Here's how the part is built. I have some questions about the finished solid (model axes, mm). A direction names the side the tool comes from. Coordinates: 2 decimals unless noted, no trailing zeros. Order: outer loops, then holes, each group sorted by start corner. A loop starts at its lowest first (then second) coordinate and runs counter-clockwise, first axis right, second up.
```python
from build123d import *

# Parameters (mm, degrees)
SKETCH1_R                                      = 17.5
BOSS_EXTRUDE1_DEPTH                            = 1.5
CUT_EXTRUDE1_DEPTH                             = 25.794152536
CUT_EXTRUDE1_DEPTH_BACK                        = 25.794152536
SKETCH6_R                                      = 0.25
SKETCH6_R_2                                    = 1
CBORE_FOR_0_SOCKET_HEAD_CAP_SCREW1_D           = 1.778
CBORE_FOR_0_SOCKET_HEAD_CAP_SCREW1_CBORE_D     = 3.175
CBORE_FOR_0_SOCKET_HEAD_CAP_SCREW1_CBORE_DEPTH = 1.016
BOSS_EXTRUDE2_START                            = -1.5
BOSS_EXTRUDE2_DEPTH                            = 1.5
FILLET1_DEPTH                                  = 1.5
CUT_EXTRUDE2_START                             = -10
SKETCH16_R                                     = 1
CUT_EXTRUDE2_DEPTH                             = 10
SKETCH17_R                                     = 6.9
CUT_EXTRUDE3_DEPTH                             = 1
FILLET2_R                                      = 0.5


with BuildPart() as part:
    # Sketch1 → Boss-Extrude1 (new body)
    with BuildSketch(Plane(origin=(0, 0, 0), x_dir=(1, 0, 0), z_dir=(0, 1, 0))):
        with Locations(Location((0, 0, 0), (0, 0, 270))):
            Circle(SKETCH1_R)
    extrude(amount=BOSS_EXTRUDE1_DEPTH)

    # Sketch6 → Cut-Extrude1 (cut, two sides: drawn at the far end of the back side and taken through both)
    with BuildSketch(Plane(origin=(0, 1.5, 0), x_dir=(1, 0, 0), z_dir=(0, 1, 0)).offset(-CUT_EXTRUDE1_DEPTH_BACK)):
        with Locations(Location((0, 12.5, 0), (0, 0, 270))):
            Circle(SKETCH6_R)
        with Locations(Location((11.591109915, 3.105828541, 0), (0, 0, 270))):
            Circle(SKETCH6_R_2)
    extrude(amount=CUT_EXTRUDE1_DEPTH + CUT_EXTRUDE1_DEPTH_BACK, mode=Mode.SUBTRACT)

    # CBORE for #0 Socket Head Cap Screw1 (through all)
    with Locations(Plane(origin=(0, 1.5, 0), x_dir=(1, 0, 0), z_dir=(0, 1, 0))):
        with Locations((0, 15), (-15, 0), (0, -15), (15, 0)):
            CounterBoreHole(CBORE_FOR_0_SOCKET_HEAD_CAP_SCREW1_D / 2, CBORE_FOR_0_SOCKET_HEAD_CAP_SCREW1_CBORE_D / 2, CBORE_FOR_0_SOCKET_HEAD_CAP_SCREW1_CBORE_DEPTH)

    # Sketch15 → Boss-Extrude2 (add)
    # profile 1 of 3: a face of its own
    with BuildSketch(Plane(origin=(0, 1.5, 0), x_dir=(1, 0, 0), z_dir=(0, 1, 0)).offset(BOSS_EXTRUDE2_START)):
        with BuildLine():
            ThreePointArc((-5.176050603, 16.717012297), (-4.139884011, 17.00327499), (-3.0880962, 17.225378424))
            Line((-3.0880962, 17.225378424), (-3.2615852, 17.702035532))
            ThreePointArc((-3.2615852, 17.702035532), (-7.18242301, 19.733545037), (-8.880129888, 15.657052506))
            ThreePointArc((-8.880129888, 15.657052506), (-8.884731942, 15.654441488), (-8.889333228, 15.651829119))
            Line((-8.889333228, 15.651829119), (-8.715826512, 15.175123334))
            ThreePointArc((-8.715826512, 15.175123334), (-7.762905696, 15.68398212), (-6.780403574, 16.133075571))
            ThreePointArc((-6.780403574, 16.133075571), (-6.498382723, 17.854159795), (-5.176050603, 16.717012297))
        make_face()
    # profile 2 of 3: a face of its own
    with BuildSketch(Plane(origin=(0, 1.5, 0), x_dir=(1, 0, 0), z_dir=(0, 1, 0)).offset(BOSS_EXTRUDE2_START)):
        with BuildLine():
            ThreePointArc((17.242700391, 2.989863415), (17.499999999, 0.00015134), (17.242752101, -2.989565186))
            Line((17.242752101, -2.989565186), (17.75, -2.989565186))
            ThreePointArc((17.75, -2.989565186), (21, 0), (17.75, 2.989565186))
            Line((17.75, 2.989565186), (17.242700391, 2.989863415))
        make_face()
        with BuildLine():
            ThreePointArc((17.972222222, 0.999614123), (19, 0), (17.972222222, -0.999614123))
            ThreePointArc((17.972222222, -0.999614123), (18, 0), (17.972222222, 0.999614123))
        make_face(mode=Mode.SUBTRACT)
    # profile 3 of 3: a face of its own
    with BuildSketch(Plane(origin=(0, 1.5, 0), x_dir=(1, 0, 0), z_dir=(0, 1, 0)).offset(BOSS_EXTRUDE2_START)):
        with BuildLine():
            ThreePointArc((-8.880129888, -15.657052506), (-6.943930938, -19.809244554), (-3.170985611, -17.210312323))
            ThreePointArc((-3.170985611, -17.210312323), (-4.180800117, -16.993260734), (-5.176050603, -16.717012297))
            ThreePointArc((-5.176050603, -16.717012297), (-6.498382723, -17.854159795), (-6.780403574, -16.133075571))
            ThreePointArc((-6.780403574, -16.133075571), (-7.758295007, -15.686263372), (-8.706903461, -15.180244798))
            Line((-8.706903461, -15.180244798), (-8.880129888, -15.657052506))
        make_face()
    extrude(amount=BOSS_EXTRUDE2_DEPTH)

    # Fillet1: read off the stored shape, not the designer's step
    # Fillet1 outline → Fillet1 (add)
    with BuildSketch(Plane(origin=(0, 0, 0), x_dir=(1, 0, 0), z_dir=(0, 1, 0))):
        with BuildLine():
            ThreePointArc((-8.889333228, 15.651829119), (-9.197952649, 15.040582781), (-9.694667487, 14.56926293))
            ThreePointArc((-9.694667487, 14.56926293), (-9.210230129, 14.880243982), (-8.715826512, 15.175123334))
            Line((-8.715826512, 15.175123334), (-8.889333228, 15.651829119))
        make_face()
        with BuildLine():
            ThreePointArc((-9.943920594, -14.400293164), (-9.235099699, -15.274689897), (-9.110766229, -16.393411442))
            ThreePointArc((-9.110766229, -16.393411442), (-9.019221723, -16.017785781), (-8.880129888, -15.657052506))
            Line((-8.880129888, -15.657052506), (-8.706903461, -15.180244798))
            ThreePointArc((-8.706903461, -15.180244798), (-9.33356259, -14.803195918), (-9.943920594, -14.400293164))
        make_face()
        with BuildLine():
            ThreePointArc((-3.0880962, 17.225378424), (-2.365537121, 17.339383902), (-1.638844908, 17.423093507))
            ThreePointArc((-1.638844908, 17.423093507), (-2.743884601, 17.637298977), (-3.558229913, 18.414369386))
            ThreePointArc((-3.558229913, 18.414369386), (-3.386909552, 18.067779761), (-3.2615852, 17.702035532))
            Line((-3.2615852, 17.702035532), (-3.0880962, 17.225378424))
        make_face()
        with BuildLine():
            ThreePointArc((17.75, 2.989565186), (18.136550606, 2.996890711), (18.520833333, 2.954442865))
            ThreePointArc((18.520833333, 2.954442865), (17.512103504, 3.453903412), (16.93287037, 4.419038472))
            ThreePointArc((16.93287037, 4.419038472), (17.102720385, 3.707688694), (17.242700391, 2.989863415))
            Line((17.242700391, 2.989863415), (17.75, 2.989565186))
        make_face()
        with BuildLine():
            ThreePointArc((17.242752101, -2.989565186), (17.102752448, -3.70754079), (16.932870371, -4.419038472))
            ThreePointArc((16.932870371, -4.419038472), (17.512103504, -3.453903412), (18.520833333, -2.954442864))
            ThreePointArc((18.520833333, -2.954442864), (18.136550606, -2.996890711), (17.75, -2.989565186))
            Line((17.75, -2.989565186), (17.242752101, -2.989565186))
        make_face()
        with BuildLine():
            ThreePointArc((-3.558229913, -18.414369386), (-2.743884601, -17.637298977), (-1.638844908, -17.423093507))
            ThreePointArc((-1.638844908, -17.423093507), (-2.407267406, -17.333639653), (-3.170985611, -17.210312323))
            ThreePointArc((-3.170985611, -17.210312323), (-3.300433079, -17.832980475), (-3.558229913, -18.414369386))
        make_face()
    extrude(amount=FILLET1_DEPTH)

    # Sketch16 → Cut-Extrude2 (cut)
    with BuildSketch(Plane(origin=(0, 1.5, 0), x_dir=(1, 0, 0), z_dir=(0, 1, 0)).offset(CUT_EXTRUDE2_START)):
        with Locations(Location((-6.15636258, 16.914467174, 0), (0, 0, 270))):
            Circle(SKETCH16_R)
        with Locations(Location((18, 0, 0), (0, 0, 270))):
            Circle(SKETCH16_R)
        with Locations(Location((-6.15636258, -16.914467174, 0), (0, 0, 270))):
            Circle(SKETCH16_R)
    extrude(amount=CUT_EXTRUDE2_DEPTH, mode=Mode.SUBTRACT)

    # Sketch17 → Cut-Extrude3 (cut)
    with BuildSketch(Plane(origin=(0, 1.5, 0), x_dir=(1, 0, 0), z_dir=(0, 1, 0))):
        with Locations(Location((0, 0, 0), (0, 0, 270))):
            Circle(SKETCH17_R)
    extrude(amount=-CUT_EXTRUDE3_DEPTH, mode=Mode.SUBTRACT)

    # Fillet2
    fillet2_edges = [part.edges().sort_by_distance(p)[0] for p in [
        (0, 0.5, -6.9),
    ]]
    fillet(fillet2_edges, radius=FILLET2_R)


solid = part.part
```
Q1. If we section it at D-D on x = 8: Write out the boundary of the cut face in (y, z).
Q2. If we section it at B-B on x = 15: Write out the boundary of the cut face in (y, z), then the cut area to 3 significant figures.
Q3. We'd pull the mould along X, two halves only. Please class faces 1 (the cylindrical face through (-16.586, 0.999, -0.07)), 2 (the flat face through (6, 1.5, 4)), 3 (the cylindrical face through (15.89, 0.24, -0.04)), 4 (the cylindrical face through (-9.24, 0.74, 15.26)): pulls with the +X half, pulls with the -X half, needs draft (parallel to the pull), parting line crosses it, or undercut.
Q4. If we section it at C-C on z = 12: Write out the boundary of the cut face in (x, y).
Q5. Will these pins go through, and if not, where does the flat tip stop? pin 1 (8 mm diameter, centred on x = -3, z = 5.5, fed in from +Y); pin 2 (1.6 mm diameter, centred on x = 0, z = 15.5, fed in from +Y).
Q6. If we section it at A-A on z = 0: Give the number of separate pieces and of enclosed holes in the cut face, then the cut area to 3 significant figures.
Q7. I need wall thicknesses on L1, parallel to Z at x = 0, y = 0.25; L2, parallel to Z at x = -14.5, y = 0.65; L3, parallel to Z at x = 15, y = 0.95. Which ranges of each line are inside material? Lowest first, please.
Q8. For faces 5 (the flat face through (1, 0, 0)), 6 (the cylindrical face through (4.66, 1.25, -5.09)), which set-ups out of +Z, -Z, +X, -X, +Y, -Y let a thin tool reach every point of the face, with its end or its side?
Reply:
1. outline: (0, -15.56) - (1.5, -15.56) - (1.5, 15.56) - (0, 15.56) - close
2. outline: (0, -9.01) - (1.5, -9.01) - (1.5, -1.59) - (0.48, -1.59) - (0.48, -0.89) - (0, -0.89) - close; (0, 0.89) - (0.48, 0.89) - (0.48, 1.59) - (1.5, 1.59) - (1.5, 9.01) - (0, 9.01) - close
2. area: 23.0 mm2
3. face 1: undercut
3. face 2: needs draft
3. face 3: undercut
3. face 4: pulls with the -X half
4. outline: (-12.74, 0) - (12.74, 0) - (12.74, 1.5) - (-12.74, 1.5) - close
5. pin 1: stops at y = 1.5
5. pin 2: stops at y = 0.48
6. separate pieces: 4
6. enclosed holes: 0
6. area: 32.9 mm2
7. L1: z = -17.5 to -15.89, -14.11 to -12.75, -12.25 to 14.11, 15.89 to 17.5
7. L2: z = -9.8 to -1.51, 1.51 to 9.8
7. L3: z = -9.01 to -1.59, 1.59 to 9.01
8. face 5: +Z, -Z, +X, -X, -Y
8. face 6: +Y
